The listing builds one solid part. Answer for the finished solid, in the listing's coordinates (mm). A direction names the side the tool comes from. Coordinates: 2 decimals unless noted, no trailing zeros. Write each loop counter-clockwise with the first axis right and the second up, starting at its lowest first coordinate (ties: lowest second). Pieces come first, ordered by that corner, then holes. Notation, with made-up numbers: M 12,-20 L 17,-20 A29 ccw 17,10 Z; hole C 58,17 d2. An arc over 180 degrees is marked long. Answer as CSV lines item,"result".
```python
from build123d import *

# Parameters (mm, degrees)
SKETCH1_W                      = 101.6
SKETCH1_H                      = 63.5
BOSS_EXTRUDE1_DEPTH            = 12.7
SKETCH2_W                      = 99.06
SKETCH2_H                      = 44.03588005
CUT_EXTRUDE1_DEPTH             = 12.7
SKETCH3_R                      = 1.5875
CUT_EXTRUDE2_DEPTH             = 3.175
CBORE_FOR_M2_SHCS1_D           = 2.4
CBORE_FOR_M2_SHCS1_CBORE_D     = 4.4
CBORE_FOR_M2_SHCS1_CBORE_DEPTH = 2


with BuildPart() as part:
    # Sketch1 → Boss-Extrude1 (new body)
    with BuildSketch(Plane.XY):
        with Locations((50.8, 31.75)):
            Rectangle(SKETCH1_W, SKETCH1_H)
    extrude(amount=BOSS_EXTRUDE1_DEPTH)

    # Sketch2 → Cut-Extrude1 (cut)
    with BuildSketch(Plane.XY.offset(12.7)):
        with Locations((50.8, 32.4134102)):
            Rectangle(SKETCH2_W, SKETCH2_H)
    extrude(amount=-CUT_EXTRUDE1_DEPTH, mode=Mode.SUBTRACT)

    # Sketch3 → Cut-Extrude2 (cut)
    with BuildSketch(Plane(origin=(0, 0, 0), x_dir=(-1, 0, 0), z_dir=(0, 0, -1))):
        with Locations((-96.8375, 4.7625)):
            Circle(SKETCH3_R)
        with Locations((-96.8375, 58.7375)):
            Circle(SKETCH3_R)
        with Locations((-4.7625, 58.7375)):
            Circle(SKETCH3_R)
        with Locations((-4.7625, 4.7625)):
            Circle(SKETCH3_R)
    extrude(amount=-CUT_EXTRUDE2_DEPTH, mode=Mode.SUBTRACT)

    # CBORE for M2 SHCS1 (through all)
    with Locations(Plane.XY.offset(12.7)):
        with Locations((96.8375, 4.7625), (96.8375, 58.7375), (4.7625, 58.7375), (4.7625, 4.71678)):
            CounterBoreHole(CBORE_FOR_M2_SHCS1_D / 2, CBORE_FOR_M2_SHCS1_CBORE_D / 2, CBORE_FOR_M2_SHCS1_CBORE_DEPTH)


solid = part.part
```
Q1. Flat-ended cylindrical pins translate along their axes: pin 1 Ø2 at (x, y) = (97, 4.5) entering from +Z; pin 2 Ø2 at (x, y) = (4.76, 4.72) entering from +Z; pin 3 Ø3 at (x, y) = (4.76, 58.74) entering from -Z (3 decimals). Find the tip coordinate at first contact, or state that the pin passes through.
Output:
pin 1,"z = 10.7"
pin 2,"through"
pin 3,"z = 3.175"
Q2. The mould has two halves that part along Y. Classify faces 4 (the flat face through (50, 0, 6)), 5 (the cylindrical face through (5.715, 3.987, 6.885)), 6 (the flat face through (101.6, 31, 6)), 7 (the flat face through (98, 4, 10.7)): pulls with the +Y half, pulls with the -Y half, needs draft (parallel to the pull), parting line crosses it, or undercut.
Output:
face 4,"pulls with the -Y half"
face 5,"undercut"
face 6,"needs draft"
face 7,"undercut"
Q3. Straight lines are drawn through the part: line 1 (Y direction, x = 46.5, z = 1.75); line 2 (X direction, y = 17.5, z = 11). For each, find the intervals that lie inside material, in ascending order.
Output:
line 1,"0 to 10.4, 54.43 to 63.5"
line 2,"0 to 1.27, 100.33 to 101.6"
Q4. Find section B-B (y = 41.5). Give the vertices of the cut face in (x, z).
Output:
outline,"M 0,0 L 1.27,0 L 1.27,12.7 L 0,12.7 Z; M 100.33,0 L 101.6,0 L 101.6,12.7 L 100.33,12.7 Z"
Q5. Find section A-A (x = 54). Give the vertices of the cut face in (y, z).
Output:
outline,"M 0,0 L 10.4,0 L 10.4,12.7 L 0,12.7 Z; M 54.43,0 L 63.5,0 L 63.5,12.7 L 54.43,12.7 Z"
Q6. Find section D-D (z = 2). Count the separate pieces of the cut face and the enclosed holes in it, and give its area (3 significant figures).
Output:
separate pieces,"1"
enclosed holes,"5"
area,"2,060 mm2"
Q7. Find section C-C (z = 6.25). Give the vertices of the cut face in (x, y).
Output:
outline,"M 0,0 L 101.6,0 L 101.6,63.5 L 0,63.5 Z; hole M 1.27,10.4 L 100.33,10.4 L 100.33,54.43 L 1.27,54.43 Z; hole C 4.76,4.72 d2.4; hole C 4.76,58.74 d2.4; hole C 96.84,4.76 d2.4; hole C 96.84,58.74 d2.4"
Q8. For faces 1 (the flat face through (54, 55, 0)), 2 (the cylindrical face through (94.64, 4.86, 11.71)), 3 (the cylindrical face through (97.182, 57.188, 1.565)), determine the directions among +Z, -Z, +X, -X, +Y, -Y from which every point of the face is accessible in a straight line to the end or side of a thin tool.
Output:
face 1,"-Z, +X, -X, +Y, -Y"
face 2,"+Z"
face 3,"-Z"
